Part model, mm, in its own coordinate system. A direction names the side the tool comes from. Coordinates: 2 decimals unless noted, no trailing zeros. Write each loop counter-clockwise with the first axis right and the second up, starting at its lowest first coordinate (ties: lowest second). Pieces come first, ordered by that corner, then holes. Notation, with made-up numbers: (-23, 9.5) - (19, 9.5) arc R18 cw to (19, 36.5) - close; hole circle Ø1 at (-23.75, -7.5). An arc over 180 degrees is marked (long way). Use a Markdown table: item, result.
```python
from build123d import *

# Parameters (mm, degrees)
SKETCH_1_W          = 40
SKETCH_1_H          = 20
EXTRUDE_1_DEPTH     = 2
SKETCH_2_W          = 10
SKETCH_2_H          = 4
EXTRUDE_2_DEPTH     = 3
CUT_EXTRUDE_1_REACH = 25.854
SKETCH_4_W          = 40
SKETCH_4_H          = 2
EXTRUDE_3_DEPTH     = 20
FILLET_1_R          = 1


with BuildPart() as part:
    # 草图1 → 凸台-拉伸1 (new body)
    with BuildSketch(Plane.XY):
        Rectangle(SKETCH_1_W, SKETCH_1_H)
    extrude(amount=EXTRUDE_1_DEPTH)

    # 草图2 → 凸台-拉伸2 (add)
    with BuildSketch(Plane.XY.offset(2)):
        Rectangle(SKETCH_2_W, SKETCH_2_H)
    extrude(amount=EXTRUDE_2_DEPTH)

    # 草图3 → 切除-拉伸1 (cut, up to next)
    with BuildSketch(Plane.XZ.offset(2), mode=Mode.PRIVATE) as cut_extrude_1_sk1:
        Polygon((-5, 5), (5, 3.236730193), (5, 5), align=None)
    cut_extrude_1_tool1 = extrude(cut_extrude_1_sk1.sketch, amount=-CUT_EXTRUDE_1_REACH, mode=Mode.PRIVATE) & part.part
    add(cut_extrude_1_tool1.solids().sort_by_distance((1.666667, -2, 4.412243))[0], mode=Mode.SUBTRACT)

    # 草图4 → 凸台-拉伸3 (add)
    with BuildSketch(Plane.XZ.offset(10)):
        with Locations((0, 1)):
            Rectangle(SKETCH_4_W, SKETCH_4_H)
    extrude(amount=EXTRUDE_3_DEPTH)

    # 圆角1
    fillet_1_edges = [part.edges().sort_by_distance(p)[0] for p in [
        (5, 0, 2),
        (0, 2, 2),
        (-5, 0, 2),
        (0, -2, 2),
    ]]
    fillet(fillet_1_edges, radius=FILLET_1_R)


solid = part.part
```
Item 1: Which spindle directions (+Z, -Z, +X, -X, +Y, -Y) get a long thin tool onto all of the face, cutting with end or side? Do faces 1 (the face through (-5, 0, 4)), 2 (the face through (20, -10, 1)), 3 (the face through (-1, 2, 4)), 4 (the face through (-1, -2, 4)). Say none if no direction does.
From the geometry:
| item | result |
|---|---|
| face 1 | +Z, -X, +Y, -Y |
| face 2 | +Z, -Z, +X, +Y, -Y |
| face 3 | +Z, +X, -X, +Y |
| face 4 | +Z, +X, -X, -Y |
Item 2: Drill centre lines: probe 1 along Z at (x, y) = (-1.5, 6.5); probe 2 along Y at (x, z) = (-2, 3.7). Where is each one in solid material? Low to high.
From the geometry:
| item | result |
|---|---|
| probe 1 | 0 to 2 |
| probe 2 | -2 to 2 |
Item 3: Band-saw the part on C-C, the plane z = 4.35. Give the cut face in (x, y), then the cut area to 3 significant figures.
From the geometry:
| item | result |
|---|---|
| outline | (-5, -2) - (-1.31, -2) - (-1.31, 2) - (-5, 2) - close |
| area | 14.7 mm^2 |
Item 4: Band-saw the part on B-B, the plane x = 0.5. Give the cut face in (y, z), then the cut area to 4 significant figures.
From the geometry:
| item | result |
|---|---|
| outline | (-30, 0) - (10, 0) - (10, 2) - (3, 2) arc R1 cw to (2, 3) - (2, 4.03) - (-2, 4.03) - (-2, 3) arc R1 cw to (-3, 2) - (-30, 2) - close |
| area | 88.55 mm^2 |
Item 5: Band-saw the part on D-D, the plane y = 5.5. Give the cut face in (x, z), then the cut area to 3 significant figures.
From the geometry:
| item | result |
|---|---|
| outline | (-20, 0) - (20, 0) - (20, 2) - (-20, 2) - close |
| area | 80.0 mm^2 |
Item 6: Drop flat-ended pins along their axis: P1, Ø2, axis at x = 0.5, z = 4, coming from the +Y side; P2, Ø2, axis at x = 9.5, y = 3.5, coming from the +Z side; P3, Ø0.6, axis at x = -1, z = 3.5, coming from the -Y side. Give the stop position or say it passes through.
From the geometry:
| item | result |
|---|---|
| P1 | y = 2 |
| P2 | z = 2 |
| P3 | y = -2 |
Item 7: Band-saw the part on A-A, the plane y = 1. Give the cut face in (x, z).
From the geometry:
| item | result |
|---|---|
| outline | (-20, 0) - (20, 0) - (20, 2) - (6, 2) arc R1 cw to (5, 3) - (5, 3.24) - (-5, 5) - (-5, 3) arc R1 cw to (-6, 2) - (-20, 2) - close |
